Can you work these out from the drawing? Everything is in mm from the part's minimum corner. A direction names the side the tool comes from. Coordinates: 2 decimals unless noted, no trailing zeros. Order: outer loops, then holes, each group sorted by start corner. A loop starts at its lowest first (then second) coordinate and runs counter-clockwise, first axis right, second up. Notation, with made-up numbers: (1.25, 72) -> (52.25, 72) arc R27 ccw to (52.25, 103) -> close; hole circle Ø8 at (0.5, -17.75). An arc over 180 degrees is marked (long way). Answer in a Markdown table with one row per item.
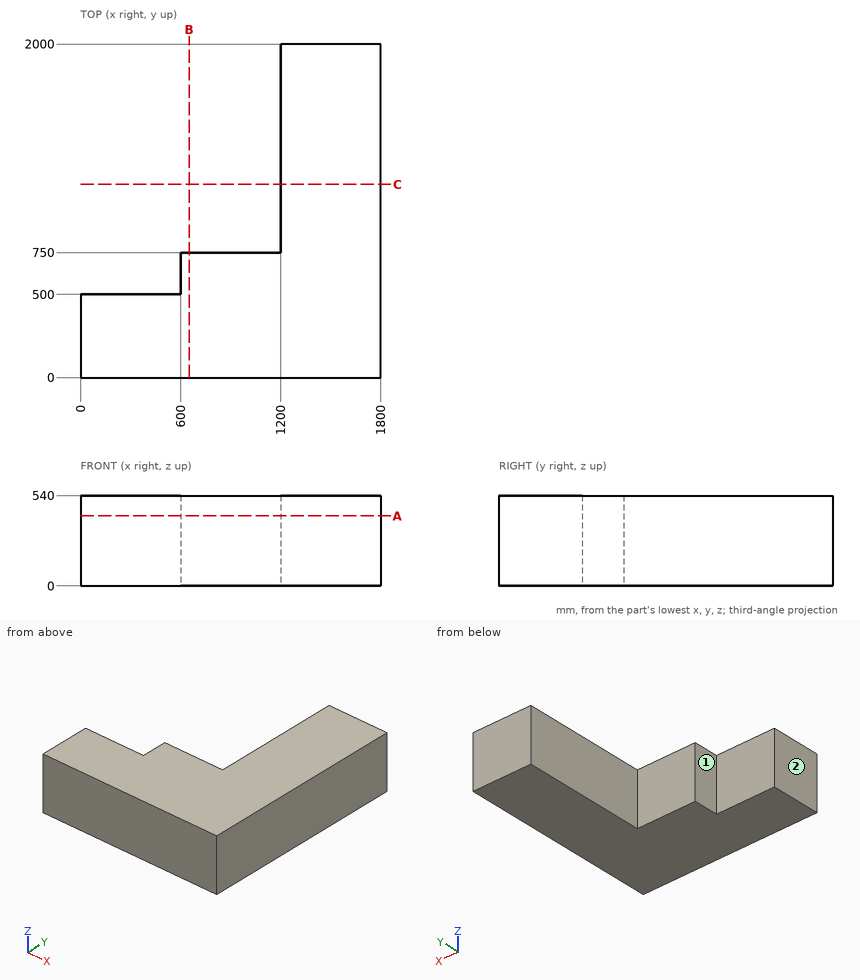
(1) On a 3-axis mill with a long thin cutter (end or side, diameter ignored), from which of +Z, -Z, +X, -X, +Y, -Y can I reach the whole of each face in a straight line? I mean the marked faces 1 and 2. Say none if no direction works.
Response values:
| item | result |
|---|---|
| face 1 | +Z, -Z, -X, +Y |
| face 2 | +Z, -Z, -X, +Y, -Y |
(2) I need wall thicknesses on line 1 (Y direction, x = 86, z = 160); line 2 (X direction, y = 1895, z = 168); line 3 (Y direction, x = 1183.5, z = 517). Which ranges of each line are inside material? Lowest first, please. Write a range as [from, to].
Response values:
| item | result |
|---|---|
| line 1 | [0, 500] |
| line 2 | [1200, 1800] |
| line 3 | [0, 750] |
(3) Suppose I cut it at C-C (y = 1159). Please give me the cut outline in (x, z), and give its area (3 significant figures).
Response values:
| item | result |
|---|---|
| outline | (1200, 0) -> (1800, 0) -> (1800, 540) -> (1200, 540) -> close |
| area | 324,000 mm2 |
(4) Will these pins go through, and if not, where does the flat tip stop? pin 1 Ø6 at (y, z) = (1047, 157.5) entering from -X; pin 2 Ø10 at (x, z) = (1043, 467) entering from +Y.
Response values:
| item | result |
|---|---|
| pin 1 | x = 1200 |
| pin 2 | y = 750 |
(5) Suppose I cut it at B-B (x = 651.5). Please give me the cut outline in (y, z).
Response values:
| item | result |
|---|---|
| outline | (0, 0) -> (750, 0) -> (750, 540) -> (0, 540) -> close |
(6) Suppose I cut it at A-A (z = 419). Please give me the cut outline in (x, y).
Response values:
| item | result |
|---|---|
| outline | (0, 0) -> (1800, 0) -> (1800, 2000) -> (1200, 2000) -> (1200, 750) -> (600, 750) -> (600, 500) -> (0, 500) -> close |
